from build123d import *

# Parameters (mm, degrees)
F2_DEPTH = 1.5


with BuildPart() as f2:
    # F1 (on Top) → F2 (new body)
    with BuildSketch(Plane.XY):
        Polygon((17.5, -75), (25.5, -75), (25.5, -58.143594), (25.5, 19.143594), (25.5, 46.856406), (25.5, 75), (-25.5, 75), (-25.5, 46.856406), (-25.5, 19.143594), (-25.5, -58.143594), (-25.5, -75), (-17.5, -75), align=None)
        Polygon((-38.5, 26.649147), (-25.5, 19.143594), (-25.5, 46.856406), (-26.5, 47.433757), align=None)
        Polygon((25.5, 46.856406), (25.5, 19.143594), (38.5, 26.649147), (26.5, 47.433757), align=None)
        Polygon((25.5, -58.143594), (25.5, -75), (17.5, -75), (17.5, -81.237604), (25.5, -85.856406), (26, -86.145082), (38, -65.360472), align=None)
        Polygon((-17.5, -81.237604), (-17.5, -75), (-25.5, -75), (-25.5, -58.143594), (-38, -65.360472), (-26, -86.145082), (-25.5, -85.856406), align=None)
    extrude(amount=F2_DEPTH)


solid = f2.part
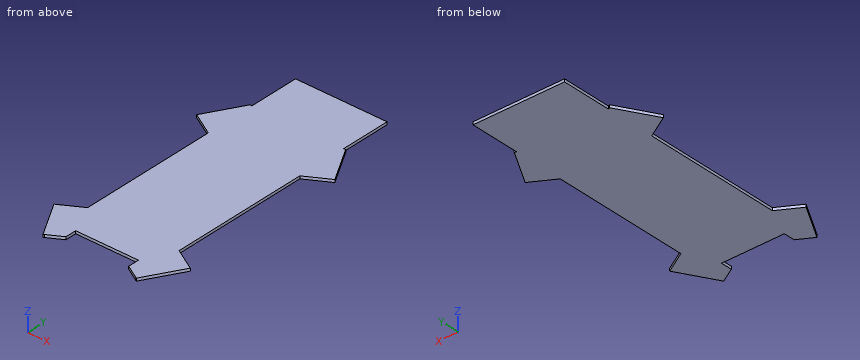
Could you check a few things on this model? Use its own coordinates, in mm. Coordinates: 2 decimals unless noted, no trailing zeros. Order: outer loops, then holes, each group sorted by start corner. A loop starts at its lowest first (then second) coordinate and runs counter-clockwise, first axis right, second up.
Q1. Suppose I cut it at D-D on x = 7. Please give me the cut outline in (y, z).
Q2. Suppose I cut it at C-C on y = -17.5. Please give me the cut outline in (x, z).
Q3. Please list where these lines run through material, in increasing order: L1, parallel to X at y = -32.5, z = 0.95; L2, parallel to Y at x = 35, z = 1.15; L3, parallel to Y at x = 7, z = 0.1.
Q4. Will these pins go through, and if not, where does the flat tip stop? pin 1 (0.8 mm diameter, centred on y = -11.5, z = 0.5, fed in from +X); pin 2 (0.8 mm diameter, centred on x = 4, z = 0.5, fed in from -Y).
Q5. Suppose I cut it at B-B on x = -33. Please give me the cut outline in (y, z), and give its area (3 significant figures).
Q6. Suppose I cut it at A-A on z = 0.4. Please give me the cut outline in (x, y), and give its area (4 significant figures).
Answer:
1. outline: (-75, 0) - (75, 0) - (75, 1.5) - (-75, 1.5) - close
2. outline: (-25.5, 0) - (25.5, 0) - (25.5, 1.5) - (-25.5, 1.5) - close
3. L1: x = -25.5 to 25.5
3. L2: y = -70.56 to -63.63, 24.63 to 32.71
3. L3: y = -75 to 75
4. pin 1: stops at x = 25.5
4. pin 2: stops at y = -75
5. outline: (-74.02, 0) - (-62.47, 0) - (-62.47, 1.5) - (-74.02, 1.5) - close; (23.47, 0) - (36.18, 0) - (36.18, 1.5) - (23.47, 1.5) - close
5. area: 36.4 mm2
6. outline: (-38.5, 26.65) - (-25.5, 19.14) - (-25.5, -58.14) - (-38, -65.36) - (-26, -86.15) - (-25.5, -85.86) - (-17.5, -81.24) - (-17.5, -75) - (17.5, -75) - (17.5, -81.24) - (25.5, -85.86) - (26, -86.15) - (38, -65.36) - (25.5, -58.14) - (25.5, 19.14) - (38.5, 26.65) - (26.5, 47.43) - (25.5, 46.86) - (25.5, 75) - (-25.5, 75) - (-25.5, 46.86) - (-26.5, 47.43) - close
6. area: 8,535 mm2
